Build history of the part. All positions in model axes, mm. A direction names the side the tool comes from. Coordinates: 2 decimals unless noted, no trailing zeros. Write each loop counter-clockwise with the first axis right and the second up, starting at its lowest first coordinate (ties: lowest second). Pieces come first, ordered by that corner, then holes.
from build123d import *

# Parameters (mm, degrees)
FILLET_1_R          = 2
CHAMFER_1_SIZE      = 2
CUT_EXTRUDE_1_DEPTH = 17
CUT_EXTRUDE_2_DEPTH = 51


with BuildPart() as part:
    # 草图1 → 旋转1 (revolve)
    with BuildSketch(Plane(origin=(0, 0, 0), x_dir=(0, 0, -1), z_dir=(1, 0, 0)), mode=Mode.PRIVATE) as revolve_1_sk:
        with BuildLine():
            Line((-275, 0), (-275, 11))
            Line((-275, 11), (-225, 11))
            Line((-225, 11), (-225, 12))
            Line((-225, 12), (-175, 12))
            Line((-175, 12), (-175, 12.5))
            Line((-175, 12.5), (-142, 12.5))
            Line((-142, 12.5), (-141.7, 12.2))
            Line((-141.7, 12.2), (-140.8, 12.2))
            ThreePointArc((-140.8, 12.2), (-140.234314575, 12.434314575), (-140, 13))
            Line((-140, 13), (-140, 15))
            Line((-140, 15), (0, 15))
            Line((0, 15), (0, 13.5))
            Line((0, 13.5), (78, 13.5))
            Line((78, 13.5), (78, 12.5))
            Line((78, 12.5), (115, 12.5))
            Line((115, 12.5), (115, 0))
            Line((115, 0), (-275, 0))
        make_face()
    revolve(revolve_1_sk.sketch.rotate(Axis((0, 0, 55.025776128), (0, 0, -1)), 90), axis=Axis((0, 0, 55.025776128), (0, 0, -1)))

    # 圆角1
    # the kernel refuses this fillet: 2 mm, written as the material it adds along each edge
    with BuildSketch(Plane(origin=(0, 0, -78), x_dir=(1, 0, 0), z_dir=(0, 1, 0))) as fillet_1_piece_1:
        with BuildLine():
            CenterArc((14.5, 1.732050808), FILLET_1_R, 180, 60)
            Line((12.5, 1.732050808), (12.46, 1.732050808))
            Line((12.46, 1.732050808), (12.46, 0))
            Line((12.46, 0), (12.5, -0.04))
            ThreePointArc((12.5, -0.04), (13, -0.04), (13.48, -0.034641016))
            Line((13.48, -0.034641016), (13.5, 0))
        make_face()
    revolve(axis=Axis((0, 0, -78), (0, 0, -1)))
    with BuildSketch(Plane(origin=(0, 0, 0), x_dir=(1, 0, 0), z_dir=(0, 1, 0))) as fillet_1_piece_2:
        with BuildLine():
            CenterArc((15.5, 1.936491673), FILLET_1_R, 180, 75.522487814)
            Line((13.5, 1.936491673), (13.46, 1.936491673))
            Line((13.46, 1.936491673), (13.46, 0))
            Line((13.46, 0), (13.5, -0.04))
            ThreePointArc((13.5, -0.04), (14.25, -0.04), (14.99, -0.038729833))
            Line((14.99, -0.038729833), (15, 0))
        make_face()
    revolve(axis=Axis((0, 0, 0), (0, 0, -1)))
    with BuildSketch(Plane(origin=(0, 0, 175), x_dir=(1, 0, 0), z_dir=(0, 1, 0))) as fillet_1_piece_3:
        with BuildLine():
            CenterArc((14, -1.322875656), FILLET_1_R, 138.590377891, 41.409622109)
            Line((12.5, 0), (12.47, 0.026457513))
            ThreePointArc((12.47, 0.026457513), (12.25, 0.04), (12, 0.04))
            Line((12, 0.04), (11.96, 0))
            Line((11.96, 0), (11.96, -1.322875656))
            Line((11.96, -1.322875656), (12, -1.322875656))
        make_face()
    revolve(axis=Axis((0, 0, 175), (0, 0, -1)))
    with BuildSketch(Plane(origin=(0, 0, 225), x_dir=(1, 0, 0), z_dir=(0, 1, 0))) as fillet_1_piece_4:
        with BuildLine():
            CenterArc((13, -1.732050808), FILLET_1_R, 120, 60)
            Line((12, 0), (11.98, 0.034641016))
            ThreePointArc((11.98, 0.034641016), (11.5, 0.04), (11, 0.04))
            Line((11, 0.04), (10.96, 0))
            Line((10.96, 0), (10.96, -1.732050808))
            Line((10.96, -1.732050808), (11, -1.732050808))
        make_face()
    revolve(axis=Axis((0, 0, 225), (0, 0, -1)))

    # 倒角1
    chamfer_1_edges = [part.edges().sort_by_distance(p)[0] for p in [
        (-12.5, 0, -115),
        (-11, 0, 275),
    ]]
    chamfer(chamfer_1_edges, length=CHAMFER_1_SIZE)

    # 草图2 → 切除-拉伸1 (cut)
    with BuildSketch(Plane(origin=(7.5, 0, 0), x_dir=(0, 0, -1), z_dir=(1, 0, 0))):
        with BuildLine():
            Line((-275, 3), (-233, 3))
            ThreePointArc((-233, 3), (-230, 0), (-233, -3))
            Line((-233, -3), (-275, -3))
            Line((-275, -3), (-275, 3))
        make_face()
    extrude(amount=CUT_EXTRUDE_1_DEPTH, mode=Mode.SUBTRACT)

    # 草图3 → 切除-拉伸2 (cut)
    with BuildSketch(Plane(origin=(9.5, 0, 0), x_dir=(0, 0, -1), z_dir=(1, 0, 0))):
        with BuildLine():
            Line((9, 4), (71, 4))
            ThreePointArc((71, 4), (75, 0), (71, -4))
            Line((71, -4), (9, -4))
            ThreePointArc((9, -4), (5, 0), (9, 4))
        make_face()
    extrude(amount=CUT_EXTRUDE_2_DEPTH, mode=Mode.SUBTRACT)


solid = part.part
(1) Slice it at D-D, the plane z = 181. List the corners of the cut face in (x, y), and give its area (3 significant figures).
(2) Probe L1, parallel to Y at x = 0.5, z = 123; L2, parallel to X at y = 8.75, z = 136.5; L3, parallel to Y at x = 11.75, z = -73. List the from-to ranges inside material, lowest first.
(3) Slice it at B-B, the plane z = 15.5. List the corners of the cut face in (x, y).
(4) 3-axis set-ups, long thin cutter, end or side, ignore diameter. For faces 1 (the cylindrical face through (-9.7, 7.4, 141.2)), 2 (the cylindrical face through (11.446, -3.604, 200.321)), 3 (the cylindrical face through (11.923, -3.755, -96.599)): which of +Z, -Z, +X, -X, +Y, -Y reach the whole face in a straight line?
(5) Flat gauge pins, fed straight in: P1, Ø3, axis at x = 11, y = -7.5, coming from the -Z side; P2, Ø2.5, axis at x = 10.5, z = -33, coming from the +Y side; P3, Ø0.9, axis at x = 9.5, z = 248, coming from the +Y side. Where does each tip first touch, or does it go through?
(6) Slice it at C-C, the plane z = 246. List the corners of the cut face in (x, y).
(7) Two-plate mould, pull along Y, no slides. Class faces 4 (the flat face through (0.1, -13.4, 140)), 5 (the flat face through (9.5, 0, -40)), 6 (the cylindrical face through (-2.38, 10.74, 249.54)): pulls with the +Y half, pulls with the -Y half, needs draft (parallel to the pull), parting line crosses it, or undercut.
Results:
1. outline: circle Ø24 at (0, 0)
1. area: 452 mm2
2. L1: y = -14.99 to 14.99
2. L2: x = -12.18 to 12.18
2. L3: y = -6.65 to -3.46, 3.46 to 6.65
3. outline: circle Ø30 at (0, 0)
4. face 1: none
4. face 2: +Z
4. face 3: -Z
5. P1: stops at z = -113.69
5. P2: stops at y = 9.83
5. P3: stops at y = 6.25
6. outline: (7.5, -3) - (7.5, 3) - (10.58, 3) arc R11 ccw (long way) to (10.58, -3) - close
7. face 4: needs draft
7. face 5: undercut
7. face 6: parting line crosses it
